Verification items for the finished model (mm, model axes). A direction names the side the tool comes from. Round coordinates to 2 decimals unless told otherwise and drop trailing zeros. Write each loop counter-clockwise with the first axis right and the second up, starting at its lowest first coordinate (ties: lowest second). Pieces come first, ordered by that corner, then holes. Notation, with made-up numbers: M -26,15.5 L 25,15.5 A15 cw 25,21.5 Z; hole C 21,24 d5. An arc over 180 degrees is marked long. One line per question, with ' | ' between items.
from build123d import *

# Parameters (mm, degrees)
SKETCH2_W          = 10.216941
SKETCH2_H          = 4
CUT_EXTRUDE1_DEPTH = 15


with BuildPart() as part:
    # Sketch1 → Revolve1 (revolve)
    with BuildSketch(Plane.XY):
        Polygon((20.35, 5.5), (12.35, 4.089384154), (12.35, -4.089384154), (20.35, -5.5), (20.35, -7.5), (8.35, -7.5), (8.35, 7.5), (20.35, 7.5), align=None)
    revolve(axis=Axis((0, -1000, 0), (0, 1, 0)))

    # Sketch2 → Cut-Extrude1 (cut)
    with BuildSketch(Plane(origin=(0, 7.5, 0), x_dir=(1, 0, 0), z_dir=(0, 1, 0))):
        with Locations((5.1084705, 0)):
            Rectangle(SKETCH2_W, SKETCH2_H)
    extrude(amount=-CUT_EXTRUDE1_DEPTH, mode=Mode.SUBTRACT)


solid = part.part
1. Mould release check, pull along Y, two halves, no side actions. Record for faces 4 (the face through (-2.786, -4.178, 12.545)), 5 (the face through (-9, 7.5, 0)), 6 (the face through (-4.411, -6.514, 19.866)): pulls with the +Y half, pulls with the -Y half, needs draft (parallel to the pull), parting line crosses it, or undercut.
Results:
face 4: undercut | face 5: pulls with the +Y half | face 6: needs draft
2. Thickness scan on line 1 (Z direction, x = 0, y = 2.5); line 2 (Z direction, x = 8.5, y = 0.25); line 3 (X direction, y = -2.5, z = -5). Record the ranges inside material, lowest first.
Results:
line 1: z = -12.35 to -8.35, 8.35 to 12.35 | line 2: z = -8.96 to -2, 2 to 8.96 | line 3: x = -11.29 to -6.69, 6.69 to 11.29
3. Tool access check on faces 1 (the face through (0, -7.5, 9)), 2 (the face through (9, 0, 2)), 3 (the face through (11.78, -0.06, -3.71)). Record the directions out of +Z, -Z, +X, -X, +Y, -Y that give a thin tool (end or side, any length) a straight path to the whole face; none if there is none.
Results:
face 1: +Z, -Z, +X, -X, -Y | face 2: +Y, -Y | face 3: none
4. Section check B-B, the plane x = 0. Record the cut outline in (y, z), then the cut area to 3 significant figures.
Results:
outline: M -7.5,-20.35 L -5.5,-20.35 L -4.09,-12.35 L 4.09,-12.35 L 5.5,-20.35 L 7.5,-20.35 L 7.5,-8.35 L -7.5,-8.35 Z; M -7.5,8.35 L 7.5,8.35 L 7.5,20.35 L 5.5,20.35 L 4.09,12.35 L -4.09,12.35 L -5.5,20.35 L -7.5,20.35 Z | area: 207 mm2
5. Section check C-C, the plane y = -3.5. Record the cut outline in (x, z), then the cut area to 3 significant figures.
Results:
outline: C 0,0 d24.7; hole M 8.11,-2 L 10.22,-2 L 10.22,2 L 8.11,2 A8.35 ccw long Z | area: 252 mm2
6. Section check A-A, the plane z = 0. Record the cut outline in (x, y).
Results:
outline: M -20.35,-7.5 L -8.35,-7.5 L -8.35,7.5 L -20.35,7.5 L -20.35,5.5 L -12.35,4.09 L -12.35,-4.09 L -20.35,-5.5 Z; M 10.22,-7.5 L 20.35,-7.5 L 20.35,-5.5 L 12.35,-4.09 L 12.35,4.09 L 20.35,5.5 L 20.35,7.5 L 10.22,7.5 Z
7. Go/stop test with flat-tipped pins: P1, Ø2.5, axis at x = 9, y = 1, coming from the +Z side; P2, Ø6, axis at y = 5, z = 8.5, coming from the -X side; P3, Ø1.5, axis at y = 2, z = 2.5, coming from the +X side. Record where each tip stops, or that it passes through.
Results:
P1: stops at z = 9.62 | P2: stops at x = -19.58 | P3: stops at x = 12.23
